Source: CAD feature listing. Evaluate the final solid. Frame: model axes, mm. Give positions to 0.01 mm unless a question says otherwise; leave off trailing zeros. Write each loop counter-clockwise with the first axis right and the second up, starting at its lowest first coordinate (ties: lowest second). Pieces come first, ordered by that corner, then holes. Notation, with made-up numbers: M 83,60.5 L 129,60.5 A34 ccw 129,97.5 Z; hole C 70.25,20 d8. An arc over 180 degrees is marked long. Return JSON: item names as keys, results as strings.
```python
from build123d import *

# Parameters (mm, degrees)
CUT_EXTRUDE2_DEPTH      = 14.290482533
CUT_EXTRUDE2_DEPTH_BACK = 14.290482533
CUT_EXTRUDE4_START      = -7.129598708
CUT_EXTRUDE4_DEPTH      = 7.129598708


# Read off the part's stored shape, not the designer's step: Cut-Extrude4
with BuildPart() as part:
    # Sketch1 → Revolve2 (revolve)
    with BuildSketch(Plane(origin=(0, 0, 0), x_dir=(1, 0, 0), z_dir=(0, 1, 0))):
        with BuildLine():
            Line((0, 0), (5.315, 0))
            Line((5.315, 0), (5.315, 5))
            ThreePointArc((5.315, 5), (3.79328092, 8.993119082), (0, 10.960769665))
            Line((0, 10.960769665), (0, 0))
        make_face()
    revolve(axis=Axis((0, 0, 0), (0, 0, -1)))

    # Sketch3 → Cut-Extrude2 (cut, two sides: drawn at the far end of the back side and taken through both)
    with BuildSketch(Plane.XY.offset(-CUT_EXTRUDE2_DEPTH_BACK)):
        Polygon((-4.924350211, -37.167719106), (-4.924350211, -2), (-4.924350211, 2), (-4.924350211, 37.167719106), (-75.259788424, 37.167719106), (-75.259788424, -37.167719106), align=None)
    extrude(amount=CUT_EXTRUDE2_DEPTH + CUT_EXTRUDE2_DEPTH_BACK, mode=Mode.SUBTRACT)

    # Cut-Extrude4 outline → Cut-Extrude4 (cut)
    with BuildSketch(Plane.XY.offset(CUT_EXTRUDE4_START)):
        with BuildLine():
            ThreePointArc((4.924350211, -2), (5.315, 0), (4.924350211, 2))
            Line((4.924350211, 2), (4.924350211, -2))
        make_face()
    extrude(amount=CUT_EXTRUDE4_DEPTH, mode=Mode.SUBTRACT)


solid = part.part
```
1) Contact query for flat-ended pins moving along their axis: pin 1 Ø1.5 at (x, z) = (2, -8) entering from -Y; pin 2 Ø4 at (y, z) = (2.5, -6.5) entering from -X; pin 3 Ø2 at (x, z) = (4, -2) entering from -Y; pin 4 Ø4 at (x, z) = (-3, -9) entering from +Y. Output: stop coordinate, or through.
Numbers:
{"pin 1": "stops at y = -4.56", "pin 2": "stops at x = -4.92", "pin 3": "stops at y = -4.39", "pin 4": "stops at y = 4.47"}
2) Cut plane A-A, the plane z = -3.25. Return the cut outline in (x, y) (3 decimals), then the cut area to 3 significant figures.
Numbers:
{"outline": "M -4.924,-2 A5.315 ccw 4.924,-2 L 4.924,2 A5.315 ccw -4.924,2 Z", "area": "86.6 mm²"}
3) Line query: line 1 (Y direction, x = -1.75, z = -9); line 2 (X direction, y = -3.75, z = -0.75); line 3 (Z direction, x = -1.75, y = 3.25). Output: solid intervals per line, ascending. Write a range as [from, to].
Numbers:
{"line 1": "y = [-3.36, 3.36]", "line 2": "x = [-3.77, 3.77]", "line 3": "z = [-9.1, 0]"}
